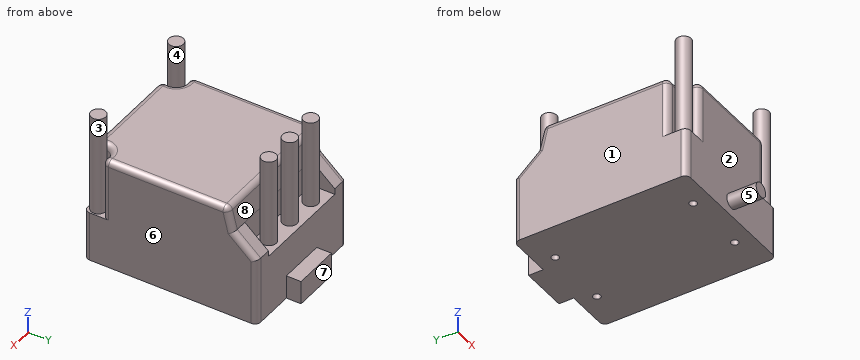
```python
from build123d import *

# Parameters (mm, degrees)
SKETCH_1_W          = 47
SKETCH_1_H          = 59
EXTRUDE_1_DEPTH     = 38
CUT_EXTRUDE_1_DEPTH = 68.25511133
SKETCH_3_W          = 35
SKETCH_3_H          = 8
CUT_EXTRUDE_2_DEPTH = 17
SKETCH_4_R          = 2.5
EXTRUDE_2_DEPTH     = 30
CUT_EXTRUDE_3_DEPTH = 21
SKETCH_6_R          = 2.5
EXTRUDE_3_DEPTH     = 34
FILLET_1_R          = 2
M3X0_51_D           = 2.5
M3X0_51_DEPTH       = 4
M3X0_51_TIP         = 0.751075774
SKETCH_10_R         = 2.5
EXTRUDE_4_DEPTH     = 10
SKETCH_11_W         = 16
SKETCH_11_H         = 8
EXTRUDE_5_DEPTH     = 5


with BuildPart() as part:
    # Эскиз1 → Бобышка-Вытянуть1 (new body)
    with BuildSketch(Plane.XY):
        Rectangle(SKETCH_1_W, SKETCH_1_H)
    extrude(amount=EXTRUDE_1_DEPTH)

    # Эскиз2 → Вырез-Вытянуть1 (cut, through all)
    with BuildSketch(Plane(origin=(23.5, 0, 0), x_dir=(0, 0, -1), z_dir=(1, 0, 0))):
        Polygon((-38, 29.5), (-38, 19.5), (-30, 21.5), (-23, 29.5), align=None)
    extrude(amount=-CUT_EXTRUDE_1_DEPTH, mode=Mode.SUBTRACT)

    # Эскиз3 → Вырез-Вытянуть2 (cut)
    with BuildSketch(Plane.XY.offset(38)):
        with Locations((0, 25.5)):
            Rectangle(SKETCH_3_W, SKETCH_3_H)
    extrude(amount=-CUT_EXTRUDE_2_DEPTH, mode=Mode.SUBTRACT)

    # Эскиз4 → Бобышка-Вытянуть2 (add)
    with BuildSketch(Plane.XY.offset(21)):
        with Locations((0, 25.5)):
            Circle(SKETCH_4_R)
        with Locations((-11, 25.5)):
            Circle(SKETCH_4_R)
        with Locations((11, 25.5)):
            Circle(SKETCH_4_R)
    extrude(amount=EXTRUDE_2_DEPTH)

    # Эскиз5 → Вырез-Вытянуть3 (cut)
    with BuildSketch(Plane.XY.offset(38)):
        with BuildLine():
            Line((-24, -26.5), (-24, -30))
            Line((-24, -30), (-20.5, -30))
            ThreePointArc((-20.5, -30), (-18.025126266, -24.025126266), (-24, -26.5))
        make_face()
        with BuildLine():
            Line((24, -26.5), (24, -30))
            Line((24, -30), (20.5, -30))
            ThreePointArc((20.5, -30), (18.025126266, -24.025126266), (24, -26.5))
        make_face()
    extrude(amount=-CUT_EXTRUDE_3_DEPTH, mode=Mode.SUBTRACT)

    # Эскиз6 → Бобышка-Вытянуть3 (add)
    with BuildSketch(Plane.XY.offset(17)):
        with Locations((-20.5, -26.5)):
            Circle(SKETCH_6_R)
        with Locations((20.5, -26.5)):
            Circle(SKETCH_6_R)
    extrude(amount=EXTRUDE_3_DEPTH)

    # Скругление1
    fillet_1_edges = [part.edges().sort_by_distance(p)[0] for p in [
        (-23.5, -2.598612181, 38),
        (-23.5, 29.5, 11.5),
        (23.5, 29.5, 11.5),
        (-23.5, 25.5, 26.5),
        (-23.5, 20.5, 34),
        (0, 19.5, 38),
        (23.5, 20.5, 34),
        (23.5, 25.5, 26.5),
        (23.5, -2.598612181, 38),
        (18.025126266, -24.025126266, 38),
        (23.5, -29.5, 8.5),
        (23.5, -24.697224362, 27.5),
        (18.697224362, -29.5, 27.5),
        (0, -29.5, 38),
        (-18.025126266, -24.025126266, 38),
        (-23.5, -29.5, 8.5),
        (-23.5, -24.697224362, 27.5),
        (-18.697224362, -29.5, 27.5),
    ]]
    fillet(fillet_1_edges, radius=FILLET_1_R)

    # Отверстие обработанное метчиком M3x0.51
    with Locations(Plane(origin=(0, 0, 0), x_dir=(-1, 0, 0), z_dir=(0, 0, -1))):
        with Locations((-11, 23.5), (11, 23.5), (11, -23.5), (-11, -23.5)):
            Hole(M3X0_51_D / 2, depth=M3X0_51_DEPTH)
            with Locations((0, 0, -(M3X0_51_DEPTH + M3X0_51_TIP / 2))):  # 118° drill point
                Cone(0, M3X0_51_D / 2, M3X0_51_TIP, mode=Mode.SUBTRACT)

    # Эскиз10 → Бобышка-Вытянуть4 (add)
    with BuildSketch(Plane.XZ.offset(29.5)):
        with Locations(Location((0, 5.26015425, 0), (0, 0, 90))):
            Circle(SKETCH_10_R)
    extrude(amount=EXTRUDE_4_DEPTH)

    # Эскиз11 → Бобышка-Вытянуть5 (add)
    with BuildSketch(Plane(origin=(0, 29.5, 0), x_dir=(1, 0, 0), z_dir=(0, 1, 0))):
        with Locations((0, -4)):
            Rectangle(SKETCH_11_W, SKETCH_11_H)
    extrude(amount=EXTRUDE_5_DEPTH)


solid = part.part
```
The listing builds one solid part. Answer for the finished solid, in the listing's coordinates (mm). Face numbers are marked on the shaded views. A direction names the side the tool comes from. Round coordinates to 2 decimals unless told otherwise and drop trailing zeros. Write each loop counter-clockwise with the first axis right and the second up, starting at its lowest first coordinate (ties: lowest second). Pieces come first, ordered by that corner, then holes. Notation, with made-up numbers: (-14.75, 35) -> (14.25, 35) arc R18 cw to (14.25, 56) -> close; hole circle Ø10 at (66, 28). An arc over 180 degrees is marked (long way). Answer as a JSON object with one key per item and string values. Group by question number.
Q1. Which of the six approach directions +Z, -Z, +X, -X, +Y, -Y give full straight-line access (tool end or side, diameter ignored) to the marked faces 4, 5, 6, 7 and 8?
Q2. Section C-C (z = 24) is taken. Count the separate pieces of the cut face and the enclosed holes in it, plus the area to 3 significant figures.
Q3. Section A-A (x = 0) is taken. Write down the section's boundary in (y, z).
Q4. Straight lines are drawn through the part: line 1 along Y through (x, z) = (-11, 2.75); line 2 along X through (y, z) = (23.5, 1.45); line 3 along Y through (x, z) = (8.5, 4.5). For each, find the intervals that lie inside material, in ascending order.
Q5. Determine the mould class of the marked faces 1, 2 and 3 for opening direction X: pulls with the +X half, pulls with the -X half, needs draft (parallel to the pull), parting line crosses it, or undercut.
Q6. Section B-B (y = 13) is taken. Write down the section's boundary in (x, z).
Q7. Each of these flat-tipped pins is pushed along its axis until it touches: pin 1 Ø5.5 at (y, z) = (32, 4.5) entering from +X; pin 2 Ø11 at (x, z) = (-0.5, 16) entering from -Y; pin 3 Ø1 at (x, y) = (-12.5, -27) entering from +Z; pin 4 Ø8 at (y, z) = (-8, 43.5) entering from -X. Where does it stop, or does it pass through?
Check values:
{
 "1": {"face 4": "+Z", "face 5": "-Y", "face 6": "+Z, -Z, +X, +Y, -Y", "face 7": "+Z, -Z, +X, -X, +Y", "face 8": "+Z, +X, -X"},
 "2": {"separate pieces": "6", "enclosed holes": "0", "area": "2,490 mm^2"},
 "3": {"outline": "(-39.5, 2.76) -> (-29.5, 2.76) -> (-29.5, 0) -> (34.5, 0) -> (34.5, 8) -> (29.5, 8) -> (29.5, 21) -> (28, 21) -> (28, 51) -> (23, 51) -> (23, 21) -> (21.5, 21) -> (21.5, 30) -> (19.88, 36.49) arc R2 ccw to (17.94, 38) -> (-27.5, 38) arc R2 ccw to (-29.5, 36) -> (-29.5, 7.76) -> (-39.5, 7.76) -> close"},
 "4": {"line 1": "-29.5 to -24.75, -22.25 to 22.25, 24.75 to 29.5", "line 2": "-23.5 to -12.25, -9.75 to 9.75, 12.25 to 23.5", "line 3": "-29.5 to 29.5"},
 "5": {"face 1": "pulls with the -X half", "face 2": "needs draft", "face 3": "undercut"},
 "6": {"outline": "(-23.5, 0) -> (23.5, 0) -> (23.5, 36) arc R2 ccw to (21.5, 38) -> (-21.5, 38) arc R2 ccw to (-23.5, 36) -> close"},
 "7": {"pin 1": "x = 22.47", "pin 2": "y = -29.5", "pin 3": "z = 38", "pin 4": "through"}
}
